Study the drawing (mm; zero at the part's minimum x, y, z) and answer. Round coordinates to 2 decimals unless told otherwise and drop trailing zeros. Loops run counter-clockwise (first coordinate to the right, second up) from the corner with the lowest first, then second, coordinate; pieces in that order, holes last. Notation, with made-up numbers: (-18.5, 18.5) - (10.5, 18.5) arc R15 cw to (10.5, 47.5) - close; hole circle Ø3 at (-40, 55.5). An arc over 180 degrees is marked (long way). One line per item, written item: value.
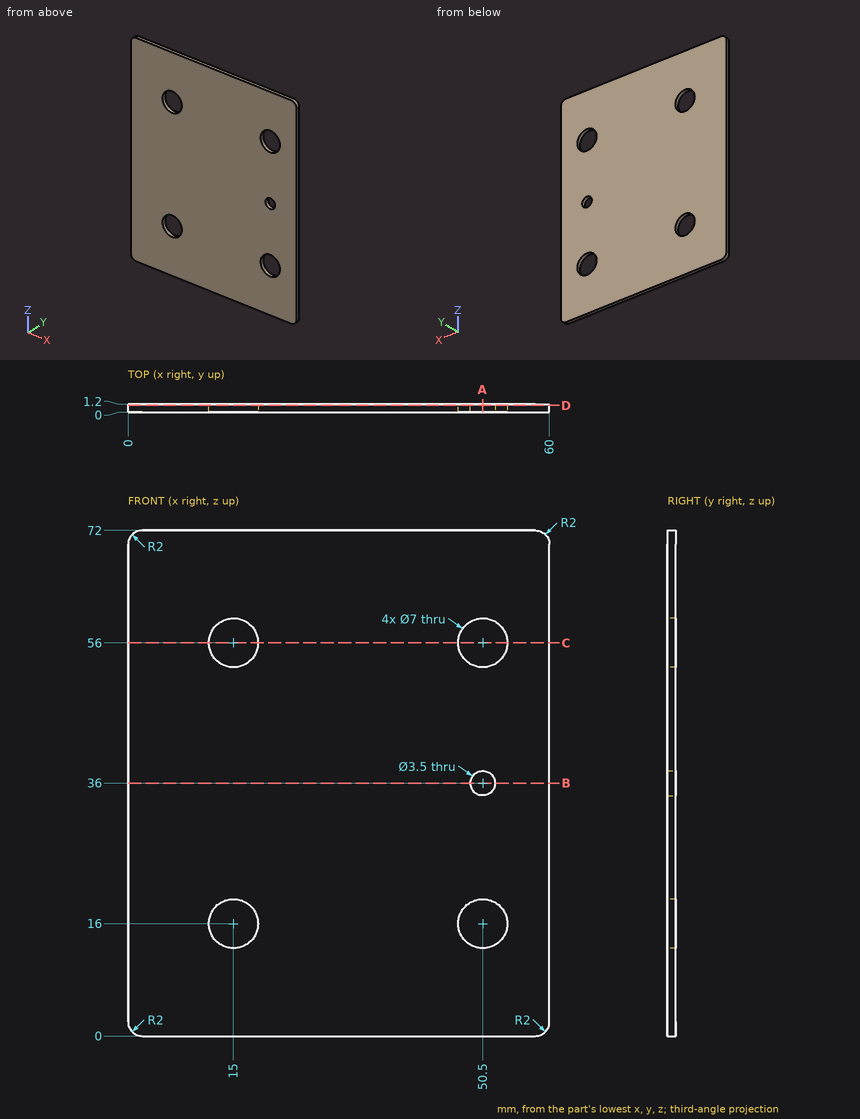
1) Consider L1, parallel to Z at x = 50.5, y = 0.8; L2, parallel to Z at x = 15, y = 0.65; L3, parallel to X at y = 0.45, z = 36. Determine where each line is inside the solid, lowest interval first.
Final values:
L1: 0 to 12.5, 19.5 to 34.25, 37.75 to 52.5, 59.5 to 72
L2: 0 to 12.5, 19.5 to 52.5, 59.5 to 72
L3: 0 to 48.75, 52.25 to 60
2) A cutting plane is placed at C-C on z = 56. Give the vertices of the cut face in (x, y), and give its area (3 significant figures).
Final values:
outline: (0, 0) - (11.5, 0) - (11.5, 1.2) - (0, 1.2) - close; (18.5, 0) - (47, 0) - (47, 1.2) - (18.5, 1.2) - close; (54, 0) - (60, 0) - (60, 1.2) - (54, 1.2) - close
area: 55.2 mm2
3) A cutting plane is placed at B-B on z = 36. Give the vertices of the cut face in (x, y).
Final values:
outline: (0, 0) - (48.75, 0) - (48.75, 1.2) - (0, 1.2) - close; (52.25, 0) - (60, 0) - (60, 1.2) - (52.25, 1.2) - close
4) A cutting plane is placed at A-A on x = 50.5. Give the vertices of the cut face in (y, z), and give its area (3 significant figures).
Final values:
outline: (0, 0) - (1.2, 0) - (1.2, 12.5) - (0, 12.5) - close; (0, 19.5) - (1.2, 19.5) - (1.2, 34.25) - (0, 34.25) - close; (0, 37.75) - (1.2, 37.75) - (1.2, 52.5) - (0, 52.5) - close; (0, 59.5) - (1.2, 59.5) - (1.2, 72) - (0, 72) - close
area: 65.4 mm2
5) A cutting plane is placed at D-D on y = 1. Give the vertices of the cut face in (x, z), and give its area (3 significant figures).
Final values:
outline: (0, 2) arc R2 ccw to (2, 0) - (58, 0) arc R2 ccw to (60, 2) - (60, 70) arc R2 ccw to (58, 72) - (2, 72) arc R2 ccw to (0, 70) - close; hole circle Ø7 at (15, 16); hole circle Ø7 at (15, 56); hole circle Ø7 at (50.5, 16); hole circle Ø7 at (50.5, 56); hole circle Ø3.5 at (50.5, 36)
area: 4,150 mm2
